Source: CAD feature listing. Evaluate the final solid. Frame: model axes, mm. Face numbers are marked on the shaded views. A direction names the side the tool comes from. Round coordinates to 2 decimals unless told otherwise and drop trailing zeros. Write each loop counter-clockwise with the first axis right and the second up, starting at its lowest first coordinate (ties: lowest second). Pieces come first, ordered by that corner, then holes.
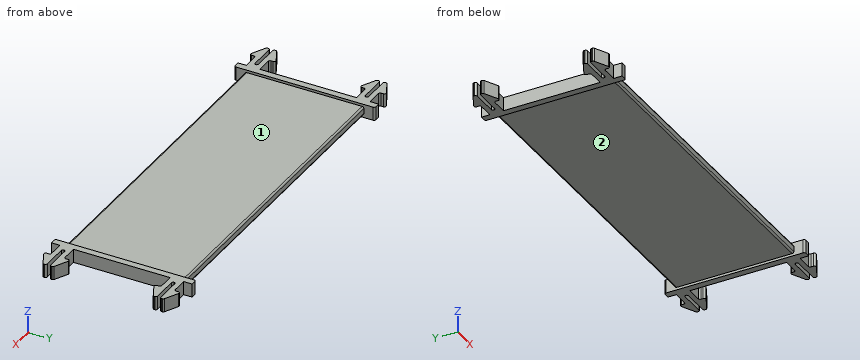
from build123d import *

# Parameters (mm, degrees)
BOSS_EXTRUDE1_DEPTH    = 8
FILLET2_R              = 1
FILLET3_R              = 1
SPLIT1_SURFACE_1_BACK  = 122.606
SPLIT1_SURFACE_1_DEPTH = 245.212
SPLIT1_SURFACE_2_BACK  = 122.606
SPLIT1_SURFACE_2_DEPTH = 245.212
LPATTERN1_START        = -8
LPATTERN1_DEPTH        = 8
SKETCH5_W              = 96
SKETCH5_H              = 8
BOSS_EXTRUDE4_DEPTH    = 73.142857143
MOVE_START             = 123.737340417
MOVE_FACE1_OUTLINE_W   = 96
MOVE_FACE1_OUTLINE_H   = 1.5
MOVE_FACE1_DEPTH       = 73.142857142
MOVE_FACE1_2_OUTLINE_W = 96
MOVE_FACE1_2_OUTLINE_H = 5
MOVE_FACE1_2_DEPTH     = 1.5
MOVE_START_2           = 195.380197559
MOVE_FACE1_3_OUTLINE_W = 96
MOVE_FACE1_3_OUTLINE_H = 5
MOVE_FACE1_3_DEPTH     = 1.5
SKETCH6_W              = 4
SKETCH6_H              = 8
BOSS_EXTRUDE3_DEPTH    = 83.142857143
FILLET4_R              = 1
FILLET5_R              = 1


# Read off the part's stored shape, not the designer's step: LPattern1, Move Face1
with BuildPart() as part:
    # Sketch1 (on Front Plane) → Boss-Extrude1 (new body)
    with BuildSketch(Plane.XY):
        Polygon((13.756813274, 188.880197559), (109.756813274, 188.880197559), (109.756813274, 196.880197559), (13.756813274, 196.880197559), (13.756813274, 201.880197559), (9.756813274, 201.880197559), (9.756813274, 196.880197559), (-0.243186726, 196.880197559), (-0.243186726, 200.880197559), (-10.243186726, 195.880197559), (-10.243186726, 193.880197559), (6.756813274, 193.880197559), (6.756813274, 191.880197559), (-10.243186726, 191.880197559), (-10.243186726, 189.880197559), (-0.243186726, 184.880197559), (-0.243186726, 188.880197559), (9.756813274, 188.880197559), (9.756813274, 183.880197559), (13.756813274, 183.880197559), align=None)
    extrude(amount=-BOSS_EXTRUDE1_DEPTH)

    # Fillet2
    fillet2_edges = [part.edges().sort_by_distance(p)[0] for p in [
        (6.756813274, 191.880197559, -4),
        (6.756813274, 193.880197559, -4),
    ]]
    fillet(fillet2_edges, radius=FILLET2_R - 0.0001)  # a hair under: the kernel refuses the full size

    # Fillet3
    fillet3_edges = [part.edges().sort_by_distance(p)[0] for p in [
        (-0.243186726, 196.880197559, -4),
        (-0.243186726, 200.880197559, -4),
        (-10.243186726, 195.880197559, -4),
        (-10.243186726, 193.880197559, -4),
        (-10.243186726, 191.880197559, -4),
        (-10.243186726, 189.880197559, -4),
        (-0.243186726, 184.880197559, -4),
        (-0.243186726, 188.880197559, -4),
    ]]
    fillet(fillet3_edges, radius=FILLET3_R)


with BuildPart() as body_2:
    # Split1: the piece behind the surface
    add(part.part)
    # Split1 surface: a surface, the sketch's curves swept straight by 245.212 mm
    with BuildLine(Plane.XY.offset(-SPLIT1_SURFACE_1_BACK), mode=Mode.PRIVATE) as split1_surface_1_path:
        Line((13.756813274, 196.880197559), (13.756813274, 188.880197559))
    split1_surface_1 = Shell.extrude(split1_surface_1_path.wire(), (0 * SPLIT1_SURFACE_1_DEPTH, 0 * SPLIT1_SURFACE_1_DEPTH, 1 * SPLIT1_SURFACE_1_DEPTH))
    split(bisect_by=split1_surface_1, keep=Keep.BOTTOM)



with BuildPart() as part_1:
    add(part.part)

    # Split1: split by a surface, the side it looks to stays
    # Split1 surface: a surface, the sketch's curves swept straight by 245.212 mm
    with BuildLine(Plane.XY.offset(-SPLIT1_SURFACE_2_BACK), mode=Mode.PRIVATE) as split1_surface_2_path:
        Line((13.756813274, 196.880197559), (13.756813274, 188.880197559))
    split1_surface_2 = Shell.extrude(split1_surface_2_path.wire(), (0 * SPLIT1_SURFACE_2_DEPTH, 0 * SPLIT1_SURFACE_2_DEPTH, 1 * SPLIT1_SURFACE_2_DEPTH))
    split(bisect_by=split1_surface_2, keep=Keep.TOP)


with BuildPart() as body_3:
    # LPattern1 outline → LPattern1 (new body)
    with BuildSketch(Plane.XY.offset(LPATTERN1_START)):
        with BuildLine():
            Line((0.756813274, 123.737340417), (9.756813274, 123.737340417))
            Line((9.756813274, 123.737340417), (9.756813274, 118.737340417))
            Line((9.756813274, 118.737340417), (13.756813274, 118.737340417))
            Line((13.756813274, 118.737340417), (13.756813274, 136.737340417))
            Line((13.756813274, 136.737340417), (9.756813274, 136.737340417))
            Line((9.756813274, 136.737340417), (9.756813274, 131.737340417))
            Line((9.756813274, 131.737340417), (0.756813274, 131.737340417))
            ThreePointArc((0.756813274, 131.737340417), (0.049706492, 132.030233635), (-0.243186726, 132.737340417))
            Line((-0.243186726, 132.737340417), (-0.243186726, 134.119306428))
            ThreePointArc((-0.243186726, 134.119306428), (-0.717455614, 134.969957236), (-1.690400321, 135.013733619))
            Line((-1.690400321, 135.013733619), (-9.690400321, 131.013733619))
            ThreePointArc((-9.690400321, 131.013733619), (-10.093837534, 130.64503754), (-10.243186726, 130.119306428))
            Line((-10.243186726, 130.119306428), (-10.243186726, 129.737340417))
            ThreePointArc((-10.243186726, 129.737340417), (-9.950293508, 129.030233635), (-9.243186726, 128.737340417))
            Line((-9.243186726, 128.737340417), (5.756813274, 128.737340417))
            ThreePointArc((5.756813274, 128.737340417), (6.463920055, 128.444447198), (6.756813274, 127.737340417))
            ThreePointArc((6.756813274, 127.737340417), (6.463920055, 127.030233635), (5.756813274, 126.737340417))
            Line((5.756813274, 126.737340417), (-9.243186726, 126.737340417))
            ThreePointArc((-9.243186726, 126.737340417), (-9.950293507, 126.444447198), (-10.243186726, 125.737340417))
            Line((-10.243186726, 125.737340417), (-10.243186726, 125.355374405))
            ThreePointArc((-10.243186726, 125.355374405), (-10.093837534, 124.829643293), (-9.690400321, 124.460947214))
            Line((-9.690400321, 124.460947214), (-1.690400321, 120.460947214))
            ThreePointArc((-1.690400321, 120.460947214), (-0.717455614, 120.504723597), (-0.243186726, 121.355374405))
            Line((-0.243186726, 121.355374405), (-0.243186726, 122.737340417))
            ThreePointArc((-0.243186726, 122.737340417), (0.049706493, 123.444447198), (0.756813274, 123.737340417))
        make_face()
    extrude(amount=LPATTERN1_DEPTH)


with BuildPart() as body_4:
    # Sketch5 → Boss-Extrude4 (new body)
    with BuildSketch(Plane(origin=(0, 196.880197559, 0), x_dir=(1, 0, 0), z_dir=(0, 1, 0))):
        with Locations((61.756813274, 4)):
            Rectangle(SKETCH5_W, SKETCH5_H)
    extrude(amount=-BOSS_EXTRUDE4_DEPTH)

    # Move Face1 outline → Move Face1 (cut)
    with BuildSketch(Plane(origin=(0, 0, 0), x_dir=(1, 0, 0), z_dir=(0, 1, 0)).offset(MOVE_START)):
        with Locations((61.756813274, 7.25)):
            Rectangle(MOVE_FACE1_OUTLINE_W, MOVE_FACE1_OUTLINE_H)
        with Locations((61.756813274, 0.75)):
            Rectangle(MOVE_FACE1_OUTLINE_W, MOVE_FACE1_OUTLINE_H)
    extrude(amount=MOVE_FACE1_DEPTH, mode=Mode.SUBTRACT)

    # Move Face1 2 outline → Move Face1 2 (cut)
    with BuildSketch(Plane(origin=(0, 0, 0), x_dir=(1, 0, 0), z_dir=(0, 1, 0)).offset(MOVE_START)):
        with Locations((61.756813274, 4)):
            Rectangle(MOVE_FACE1_2_OUTLINE_W, MOVE_FACE1_2_OUTLINE_H)
    extrude(amount=MOVE_FACE1_2_DEPTH, mode=Mode.SUBTRACT)

    # Move Face1 3 outline → Move Face1 3 (cut)
    with BuildSketch(Plane(origin=(0, 0, 0), x_dir=(1, 0, 0), z_dir=(0, 1, 0)).offset(MOVE_START_2)):
        with Locations((61.756813274, 4)):
            Rectangle(MOVE_FACE1_3_OUTLINE_W, MOVE_FACE1_3_OUTLINE_H)
    extrude(amount=MOVE_FACE1_3_DEPTH, mode=Mode.SUBTRACT)


with BuildPart() as body_2_1:
    add(body_2.part)

    add(body_3.part)  # Boss-Extrude3 merges body 3

    add(body_4.part)  # Boss-Extrude3 merges body 4
    # Sketch6 → Boss-Extrude3 (add)
    with BuildSketch(Plane(origin=(0, 201.880197559, 0), x_dir=(1, 0, 0), z_dir=(0, 1, 0))):
        with Locations((11.756813274, 4)):
            Rectangle(SKETCH6_W, SKETCH6_H)
    extrude(amount=-BOSS_EXTRUDE3_DEPTH)

    # Fillet4
    fillet4_edges = [body_2_1.edges().sort_by_distance(p)[0] for p in [
        (13.756813274, 118.737340417, -4),
        (13.756813274, 201.880197559, -4),
    ]]
    fillet(fillet4_edges, radius=FILLET4_R)

    # Mirror1: body 2 across plane


with BuildPart() as body_2_2:
    add(body_2_1.part)
    add(body_2_1.part.mirror(Plane(origin=(109.756813274, 27.404583786, 0), x_dir=(0, 0, 1), z_dir=(1, 0, 0))))

    # Fillet5
    fillet5_edges = [body_2_2.edges().sort_by_distance(p)[0] for p in [
        (109.756813274, 195.380197559, -1.5),
        (109.756813274, 195.380197559, -6.5),
        (109.756813274, 125.237340417, -6.5),
        (109.756813274, 125.237340417, -1.5),
    ]]
    fillet(fillet5_edges, radius=FILLET5_R)


solid = body_2_2.part
1) Section query B-B on y = 174. Return the cut outline in (x, z), then the cut area to 3 significant figures.
Taken from the geometry:
outline: (9.76, -8) - (13.76, -8) - (13.76, -6.5) - (205.76, -6.5) - (205.76, -8) - (209.76, -8) - (209.76, 0) - (205.76, 0) - (205.76, -1.5) - (13.76, -1.5) - (13.76, 0) - (9.76, 0) - close
area: 1,020 mm2
2) Reachability of the marked faces 1 and 2 from +Z, -Z, +X, -X, +Y, -Y: full face, straight path, thin tool, end or side. Return the list, or none.
Taken from the geometry:
face 1: +Z, +Y, -Y
face 2: -Z, +Y, -Y
3) Material intervals for line 1 (Y direction, x = 215, z = -5.5); line 2 (X direction, y = 183.5, z = -1); line 3 (Z direction, x = 69.5, y = 138.5), sorted ascending.
Taken from the geometry:
line 1: y = 123.74 to 126.74, 128.74 to 131.74, 188.88 to 191.88, 193.88 to 196.88
line 2: x = 9.76 to 13.76, 205.76 to 209.76
line 3: z = -6.5 to -1.5
4) Contact query for flat-ended pins moving along their axis: P1, Ø4, axis at y = 141.5, z = -1.5, coming from the +X side; P2, Ø2, axis at x = 36.5, y = 161, coming from the +Z side; P3, Ø3.5, axis at x = 72.5, z = -3.5, coming from the -Y side. Output: stop coordinate, or through.
Taken from the geometry:
P1: stops at x = 209.76
P2: stops at z = -1.5
P3: stops at y = 125.24
5) Section query A-A on x = 123. Return the cut outline in (y, z), then the cut area to 3 significant figures.
Taken from the geometry:
outline: (125.24, -5.5) arc R1 ccw to (126.24, -6.5) - (194.38, -6.5) arc R1 ccw to (195.38, -5.5) - (195.38, -2.5) arc R1 ccw to (194.38, -1.5) - (126.24, -1.5) arc R1 ccw to (125.24, -2.5) - close
area: 350 mm2
